from build123d import *

# Parameters (mm, degrees)
SKETCH_1_R          = 16.15
EXTRUDE_1_DEPTH     = 3
SKETCH_2_R          = 1.45
CUT_EXTRUDE_1_DEPTH = 5
FILLET_1_R          = 3
CUT_EXTRUDE_2_DEPTH = 52.529117982
FILLET_2_R          = 2


with BuildPart() as part:
    # 草图1 → 凸台-拉伸1 (new body)
    with BuildSketch(Plane.XY):
        with BuildLine():
            Line((-22, 0), (-22, -46.5))
            Line((-22, -46.5), (22, -46.5))
            Line((22, -46.5), (22, 0))
            ThreePointArc((22, 0), (0, 22), (-22, 0))
        make_face()
        Circle(SKETCH_1_R, mode=Mode.SUBTRACT)
    extrude(amount=EXTRUDE_1_DEPTH)

    # 草图2 → 切除-拉伸1 (cut)
    with BuildSketch(Plane.XY.offset(3)):
        with Locations((0, -41.5)):
            Circle(SKETCH_2_R)
        with Locations((17, -41.5)):
            Circle(SKETCH_2_R)
        with Locations((-17, -41.5)):
            Circle(SKETCH_2_R)
        with Locations((0, 18.95)):
            Circle(SKETCH_2_R)
        with Locations((18.95, 0)):
            Circle(SKETCH_2_R)
        with Locations((0, -18.95)):
            Circle(SKETCH_2_R)
        with Locations((-18.95, 0)):
            Circle(SKETCH_2_R)
        with Locations((-17, -29.5)):
            Circle(SKETCH_2_R)
        with Locations((17, -29.5)):
            Circle(SKETCH_2_R)
    extrude(amount=-CUT_EXTRUDE_1_DEPTH, mode=Mode.SUBTRACT)

    # 圆角1
    fillet_1_edges = [part.edges().sort_by_distance(p)[0] for p in [
        (22, -46.5, 1.5),
        (-22, -46.5, 1.5),
    ]]
    fillet(fillet_1_edges, radius=FILLET_1_R)

    # 草图3 → 切除-拉伸2 (cut, through all)
    with BuildSketch(Plane(origin=(0, 0, 0), x_dir=(-1, 0, 0), z_dir=(0, 0, -1))):
        Polygon((-17.217121795, -16.002095348), (-3, -20.95), (-3, -39.5), (-11.462229393, -39.5), align=None)
        Polygon((17.217121795, -16.002095348), (3, -20.95), (3, -39.5), (11.462229393, -39.5), align=None)
    extrude(amount=-CUT_EXTRUDE_2_DEPTH, mode=Mode.SUBTRACT)

    # 圆角2
    fillet_2_edges = [part.edges().sort_by_distance(p)[0] for p in [
        (11.462229393, -39.5, 1.5),
        (17.217121795, -16.002095348, 1.5),
        (3, -20.95, 1.5),
        (3, -39.5, 1.5),
        (-3, -39.5, 1.5),
        (-3, -20.95, 1.5),
        (-17.217121795, -16.002095348, 1.5),
        (-11.462229393, -39.5, 1.5),
    ]]
    fillet(fillet_2_edges, radius=FILLET_2_R)


solid = part.part
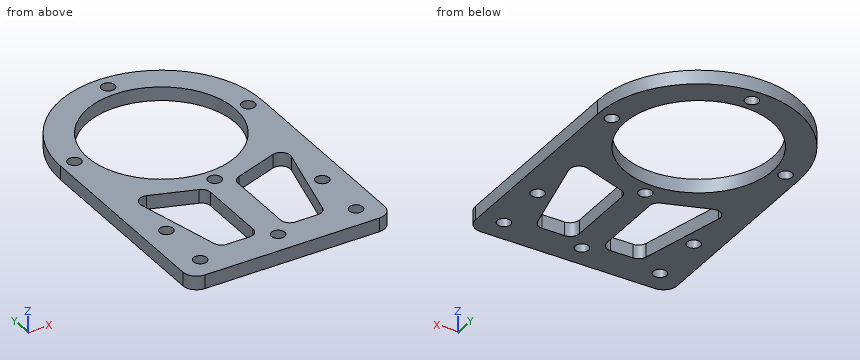
Read the model definition and answer for the solid it produces. Units are mm, in the model's axes. Round coordinates to 2 decimals unless told otherwise and drop trailing zeros. Write each loop counter-clockwise with the first axis right and the second up, starting at its lowest first coordinate (ties: lowest second). Pieces come first, ordered by that corner, then holes. Notation, with made-up numbers: (75, 88.25) - (91, 88.25) arc R26 ccw to (91, 126.25) - close; hole circle Ø9 at (-36.5, 36.25). An arc over 180 degrees is marked (long way). Use a Markdown table: item, result.
(1) The part is cut by section C-C (y = -26.5). Write down the section's boundary in (x, z).
Reported:
| item | result |
|---|---|
| outline | (-22, 0) - (-14.65, 0) - (-14.65, 3) - (-22, 3) - close; (-3, 0) - (3, 0) - (3, 3) - (-3, 3) - close; (14.65, 0) - (22, 0) - (22, 3) - (14.65, 3) - close |
(2) The part is cut by section A-A (x = 0). Write down the section's boundary in (y, z).
Reported:
| item | result |
|---|---|
| outline | (-46.5, 0) - (-42.95, 0) - (-42.95, 3) - (-46.5, 3) - close; (-40.05, 0) - (-20.4, 0) - (-20.4, 3) - (-40.05, 3) - close; (-17.5, 0) - (-16.15, 0) - (-16.15, 3) - (-17.5, 3) - close; (16.15, 0) - (17.5, 0) - (17.5, 3) - (16.15, 3) - close; (20.4, 0) - (22, 0) - (22, 3) - (20.4, 3) - close |
(3) The part is cut by section B-B (z = 2.4). State how many separate pieces and enclosed holes the cut face has, then the cut area to 3 significant figures.
Reported:
| item | result |
|---|---|
| separate pieces | 1 |
| enclosed holes | 12 |
| area | 1,470 mm2 |
(4) Straight lines are drawn through the part: line 1 along Y through (x, z) = (0, 1.1); line 2 along X through (y, z) = (-31, 1.05); line 3 along Y through (x, z) = (-17, 1.75). For each, find the intervals that lie inside material, in ascending order. Write a range as [from, to].
Reported:
| item | result |
|---|---|
| line 1 | [-46.5, -42.95], [-40.05, -20.4], [-17.5, -16.15], [16.15, 17.5], [20.4, 22] |
| line 2 | [-22, -13.54], [-3, 3], [13.54, 22] |
| line 3 | [-46.5, -42.95], [-40.05, -30.95], [-28.05, 13.96] |
(5) The part is cut by section D-D (x = -13). Write down the section's boundary in (y, z).
Reported:
| item | result |
|---|---|
| outline | (-46.5, 0) - (-33.22, 0) - (-33.22, 3) - (-46.5, 3) - close; (-17.47, 0) - (-9.58, 0) - (-9.58, 3) - (-17.47, 3) - close; (9.58, 0) - (17.75, 0) - (17.75, 3) - (9.58, 3) - close |
(6) Each of these flat-tipped pins is pushed along its axis until it touches: pin 1 Ø1.5 at (x, z) = (7, 1.5) entering from +Y; pin 2 Ø2.5 at (x, y) = (0, -41.5) entering from -Z; pin 3 Ø0.9 at (x, z) = (-8.5, 1) entering from +Y. Where does it stop, or does it pass through?
Reported:
| item | result |
|---|---|
| pin 1 | y = 21.09 |
| pin 2 | through |
| pin 3 | y = 20.47 |
